from build123d import *

# Parameters (mm, degrees)
SKETCH1_W               = 48.8
SKETCH1_H               = 55
BOSS_EXTRUDE1_DEPTH     = 3
SKETCH2_W               = 4.5
SKETCH2_H               = 4.5
BOSS_EXTRUDE2_DEPTH     = 13.8
FILLET1_R               = 5
FILLET2_START           = -27.5
FILLET2_DEPTH           = 4.5
MIRROR4_COPY_1_SKETCH_W = 4.5
MIRROR4_COPY_1_SKETCH_H = 4.5
MIRROR4_COPY_1_DEPTH    = 13.8
FILLET3_R               = 5
FILLET4_START           = -27.5
FILLET4_DEPTH           = 4.5
FILLET5_R               = 5
FILLET6_START           = 23
FILLET6_DEPTH           = 4.5
FILLET7_R               = 5
FILLET8_START           = 23
FILLET8_DEPTH           = 4.5


with BuildPart() as part:
    # Sketch1 → Boss-Extrude1 (new body)
    with BuildSketch(Plane(origin=(0, 0, 0), x_dir=(1, 0, 0), z_dir=(0, 1, 0))):
        Rectangle(SKETCH1_W, SKETCH1_H)
    extrude(amount=BOSS_EXTRUDE1_DEPTH)

    # Sketch2 → Boss-Extrude2 (add)
    with BuildSketch(Plane(origin=(0, 3, 0), x_dir=(1, 0, 0), z_dir=(0, 1, 0))):
        with Locations((-22.15, 25.25)):
            Rectangle(SKETCH2_W, SKETCH2_H)
    boss_extrude2 = extrude(amount=BOSS_EXTRUDE2_DEPTH)

    # Sketch11 → M3x0.5 Tapped Hole1 (revolve, cut)
    with BuildSketch(Plane(origin=(-22.15, 16.8, -25.25), x_dir=(0, 0, 1), z_dir=(1, 0, 0))):
        Polygon((0, 0), (0, 7.751075774), (1.25, 7), (1.25, 0), align=None)
    m3x0_5_tapped_hole1 = revolve(axis=Axis((-22.15, 23.15, -25.25), (0, -1, 0)), mode=Mode.SUBTRACT)

    # Sketch13 → M3 Clearance Hole1 (revolve, cut)
    with BuildSketch(Plane(origin=(-17.5, 3, -16.7), x_dir=(0, 0, 1), z_dir=(1, 0, 0))):
        Polygon((0, 0), (0, 9.521463052), (1.7, 8.5), (1.7, 0), align=None)
    m3_clearance_hole1 = revolve(axis=Axis((-17.5, 9.35, -16.7), (0, -1, 0)), mode=Mode.SUBTRACT)

    # Fillet1
    fillet1_edges = [part.edges().sort_by_distance(p)[0] for p in [
        (-22.15, 3, -23),
    ]]
    fillet(fillet1_edges, radius=FILLET1_R)

    # Fillet2: read off the stored shape, not the designer's step
    # Fillet2 outline → Fillet2 (add)
    with BuildSketch(Plane.XY.offset(FILLET2_START)):
        with BuildLine():
            ThreePointArc((-14.9, 3), (-18.435533906, 4.464466094), (-19.9, 8))
            Line((-19.9, 8), (-19.9, 3))
            Line((-19.9, 3), (-14.9, 3))
        make_face()
    extrude(amount=FILLET2_DEPTH)

    # Mirror3: Boss-Extrude2, M3x0.5 Tapped Hole1, M3 Clearance Hole1 across plane
    add(boss_extrude2.mirror(Plane(origin=(0, 0, 0), x_dir=(0, 0, 1), z_dir=(1, 0, 0))))
    add(m3x0_5_tapped_hole1.mirror(Plane(origin=(0, 0, 0), x_dir=(0, 0, 1), z_dir=(1, 0, 0))), mode=Mode.SUBTRACT)
    add(m3_clearance_hole1.mirror(Plane(origin=(0, 0, 0), x_dir=(0, 0, 1), z_dir=(1, 0, 0))), mode=Mode.SUBTRACT)

    # Mirror4: Boss-Extrude2, M3x0.5 Tapped Hole1, M3 Clearance Hole1 across plane
    add(boss_extrude2.mirror(Plane.XY))
    add(m3x0_5_tapped_hole1.mirror(Plane.XY), mode=Mode.SUBTRACT)
    add(m3_clearance_hole1.mirror(Plane.XY), mode=Mode.SUBTRACT)

    # Mirror4 copy 1 sketch → Mirror4 copy 1 (add)
    with BuildSketch(Plane(origin=(0, 3, 0), x_dir=(-1, 0, 0), z_dir=(0, 1, 0))):
        with Locations((-22.15, 25.25)):
            Rectangle(MIRROR4_COPY_1_SKETCH_W, MIRROR4_COPY_1_SKETCH_H)
    extrude(amount=MIRROR4_COPY_1_DEPTH)

    # Mirror4 copy 2 sketch → Mirror4 copy 2 (revolve, cut)
    with BuildSketch(Plane(origin=(22.15, 16.8, 25.25), x_dir=(0, 0, -1), z_dir=(-1, 0, 0))):
        Polygon((0, 0), (0, 7.751075774), (1.25, 7), (1.25, 0), align=None)
    revolve(axis=Axis((22.15, 23.15, 25.25), (0, -1, 0)), mode=Mode.SUBTRACT)

    # Mirror4 copy 3 sketch → Mirror4 copy 3 (revolve, cut)
    with BuildSketch(Plane(origin=(17.5, 3, 16.7), x_dir=(0, 0, -1), z_dir=(-1, 0, 0))):
        Polygon((0, 0), (0, 9.521463052), (1.7, 8.5), (1.7, 0), align=None)
    revolve(axis=Axis((17.5, 9.35, 16.7), (0, -1, 0)), mode=Mode.SUBTRACT)

    # Fillet3
    fillet3_edges = [part.edges().sort_by_distance(p)[0] for p in [
        (22.15, 3, -23),
    ]]
    fillet(fillet3_edges, radius=FILLET3_R)

    # Fillet4: read off the stored shape, not the designer's step
    # Fillet4 outline → Fillet4 (add)
    with BuildSketch(Plane.XY.offset(FILLET4_START)):
        with BuildLine():
            Line((19.9, 3), (19.9, 8))
            ThreePointArc((19.9, 8), (18.435533906, 4.464466094), (14.9, 3))
            Line((14.9, 3), (19.9, 3))
        make_face()
    extrude(amount=FILLET4_DEPTH)

    # Fillet5
    fillet5_edges = [part.edges().sort_by_distance(p)[0] for p in [
        (22.15, 3, 23),
    ]]
    fillet(fillet5_edges, radius=FILLET5_R)

    # Fillet6: read off the stored shape, not the designer's step
    # Fillet6 outline → Fillet6 (add)
    with BuildSketch(Plane.XY.offset(FILLET6_START)):
        with BuildLine():
            Line((19.9, 3), (19.9, 8))
            ThreePointArc((19.9, 8), (18.435533906, 4.464466094), (14.9, 3))
            Line((14.9, 3), (19.9, 3))
        make_face()
    extrude(amount=FILLET6_DEPTH)

    # Fillet7
    fillet7_edges = [part.edges().sort_by_distance(p)[0] for p in [
        (-22.15, 3, 23),
    ]]
    fillet(fillet7_edges, radius=FILLET7_R)

    # Fillet8: read off the stored shape, not the designer's step
    # Fillet8 outline → Fillet8 (add)
    with BuildSketch(Plane.XY.offset(FILLET8_START)):
        with BuildLine():
            ThreePointArc((-14.9, 3), (-18.435533906, 4.464466094), (-19.9, 8))
            Line((-19.9, 8), (-19.9, 3))
            Line((-19.9, 3), (-14.9, 3))
        make_face()
    extrude(amount=FILLET8_DEPTH)


solid = part.part
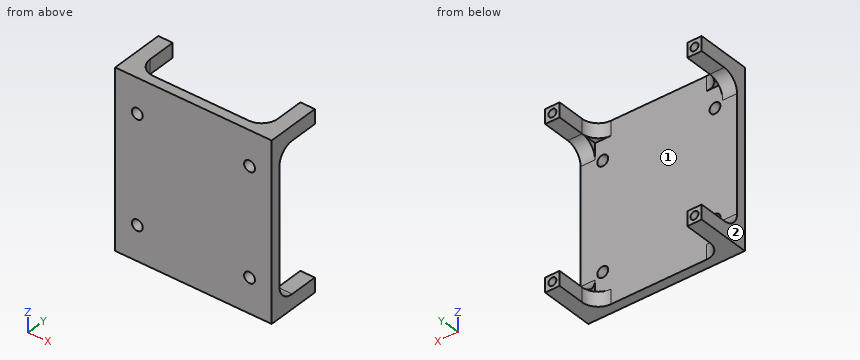
Geometry: final body of the model. Coordinates: model frame, mm. Face numbers are marked on the shaded views. A direction names the side the tool comes from. Coordinates: 2 decimals unless noted, no trailing zeros. Order: outer loops, then holes, each group sorted by start corner. A loop starts at its lowest first (then second) coordinate and runs counter-clockwise, first axis right, second up.
(1) Section query C-C (x = -7.5). Return the cut outline in (y, z), plus the area to 3 significant figures.
(2) Access query for the marked faces 1 and 2. Directions: +Z, -Z, +X, -X, +Y, -Y. A direction counts if a zero-diameter tool reaches every point of the face in a straight line with its end or side. Return the directions, or none.
(3) Material intervals for probe 1 along Z at (x, y) = (-17.5, 1.8); probe 2 along X at (y, z) = (0.95, -16.7); probe 3 along X at (y, z) = (15.75, -25.25), sorted ascending.
(4) First-contact query: pin 1 (2 mm diameter, centred on x = -22.15, z = -25.25, fed in from -Y); pin 2 (5.5 mm diameter, centred on x = -17.5, z = 16.7, fed in from +Y); pin 3 (1.5 mm diameter, centred on x = -16.5, y = 5.5, fed in from +Z). Flat tips, straight axial feed; report the tip coordinate or a pass-through.
(5) Section query A-A (y = 14.5). Return the cut outline in (x, z).
(6) Section query D-D (z = -13). Return the cut outline in (x, y).
(7) Section query B-B (x = 17.5). Return the cut outline in (y, z), plus the area to 3 significant figures.
Solution:
1. outline: (0, -27.5) - (3, -27.5) - (3, 27.5) - (0, 27.5) - close
1. area: 165 mm2
2. face 1: +Y
2. face 2: +Z, -Z, -X, +Y, -Y
3. probe 1: z = -27.5 to -18.4, -15 to 15, 18.4 to 27.5
3. probe 2: x = -24.4 to -19.2, -15.8 to 15.8, 19.2 to 24.4
3. probe 3: x = -24.4 to -23.4, -20.9 to -19.9, 19.9 to 20.9, 23.4 to 24.4
4. pin 1: stops at y = 0
4. pin 2: stops at y = 3
4. pin 3: passes through
5. outline: (-24.4, -27.5) - (-19.9, -27.5) - (-19.9, -23) - (-24.4, -23) - close; (-24.4, 23) - (-19.9, 23) - (-19.9, 27.5) - (-24.4, 27.5) - close; (19.9, -27.5) - (24.4, -27.5) - (24.4, -23) - (19.9, -23) - close; (19.9, 23) - (24.4, 23) - (24.4, 27.5) - (19.9, 27.5) - close; hole circle Ø2.5 at (-22.15, -25.25); hole circle Ø2.5 at (-22.15, 25.25); hole circle Ø2.5 at (22.15, -25.25); hole circle Ø2.5 at (22.15, 25.25)
6. outline: (-24.4, 0) - (24.4, 0) - (24.4, 3) - (-24.4, 3) - close
7. outline: (0, -27.5) - (3.73, -27.5) - (3.73, -23) - (3, -23) - (3, -18.4) - (0, -18.4) - close; (0, -15) - (3, -15) - (3, 15) - (0, 15) - close; (0, 18.4) - (3, 18.4) - (3, 23) - (3.73, 23) - (3.73, 27.5) - (0, 27.5) - close
7. area: 151 mm2
